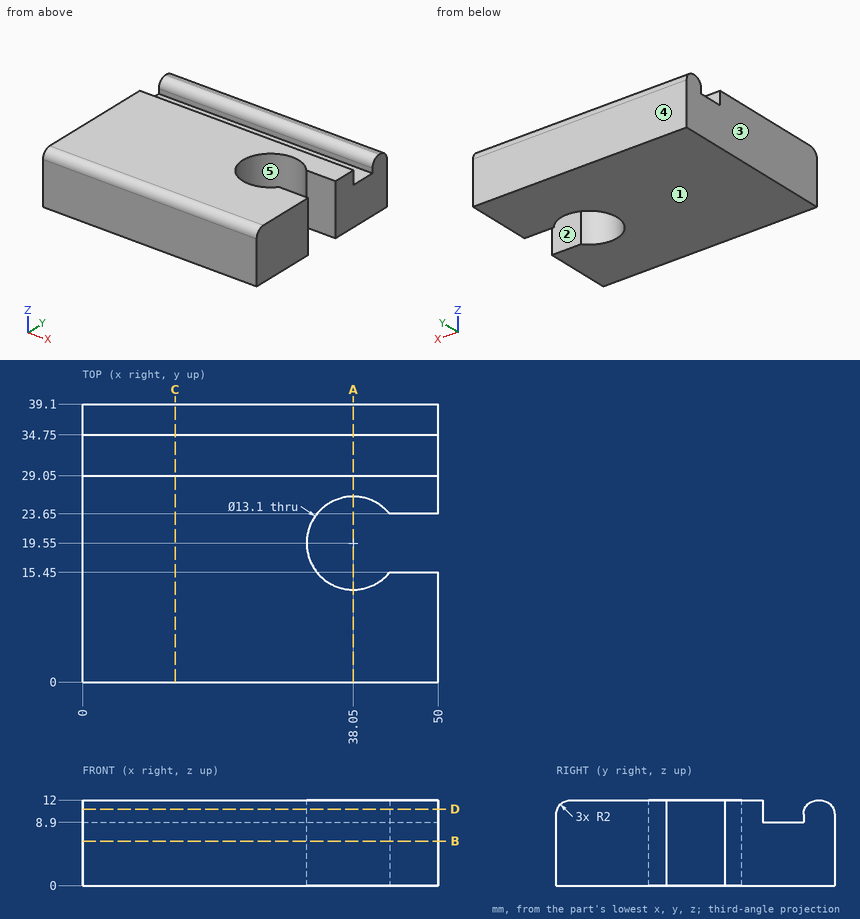
Answer from the drawing. Dimensions are ordinates in mm from the lowest x, y and z of the part. A direction names the side the tool comes from. Round coordinates to 2 decimals unless told otherwise and drop trailing zeros. Loops run counter-clockwise (first coordinate to the right, second up) from the corner with the lowest first, then second, coordinate; pieces in that order, holes last.
1) Given P1, Ø1, axis at x = 8, y = 31, coming from the +Z side, flat-ended and moving along its own axis, determine where the tip first touches the part or whether it passes through.
Outcome:
P1: stops at z = 8.9
2) A cutting plane is placed at C-C on x = 13. Determine the outline of the cut face in (y, z).
Outcome:
outline: (0, 0) - (39.1, 0) - (39.1, 10) arc R2 ccw to (37.1, 12) - (36.75, 12) arc R2 ccw to (34.75, 10) - (34.75, 8.9) - (29.05, 8.9) - (29.05, 12) - (2, 12) arc R2 ccw to (0, 10) - close
3) For the marked faces 1 and 2, determine the directions among +Z, -Z, +X, -X, +Y, -Y from which every point of the face is accessible in a straight line to the end or side of a thin tool.
Outcome:
face 1: -Z, +X, -X, +Y, -Y
face 2: +Z, -Z, +X
4) A cutting plane is placed at D-D on z = 10.75. Determine the outline of the cut face in (x, y).
Outcome:
outline: (0, 0.15) - (50, 0.15) - (50, 15.45) - (43.16, 15.45) arc R6.55 cw (long way) to (43.16, 23.65) - (50, 23.65) - (50, 29.05) - (0, 29.05) - close; (0, 34.9) - (50, 34.9) - (50, 38.95) - (0, 38.95) - close
5) For a pull along X with two mould halves and no side action, classify the marked faces 3, 4 and 5 as released by +X, released by -X, zero draft, split by the parting line, or undercut.
Outcome:
face 3: released by -X
face 4: zero draft
face 5: undercut
6) A cutting plane is placed at A-A on x = 38.05. Determine the outline of the cut face in (y, z).
Outcome:
outline: (0, 0) - (13, 0) - (13, 12) - (2, 12) arc R2 ccw to (0, 10) - close; (26.1, 0) - (39.1, 0) - (39.1, 10) arc R2 ccw to (37.1, 12) - (36.75, 12) arc R2 ccw to (34.75, 10) - (34.75, 8.9) - (29.05, 8.9) - (29.05, 12) - (26.1, 12) - close
7) Consider line 1 (Y direction, x = 38.05, z = 3.5); line 2 (Y direction, x = 27.5, z = 9.75); line 3 (X direction, y = 19.55, z = 3). Determine where each line is inside the solid, lowest interval first.
Outcome:
line 1: y = 0 to 13, 26.1 to 39.1
line 2: y = 0 to 29.05, 34.75 to 39.1
line 3: x = 0 to 31.5
8) A cutting plane is placed at B-B on z = 6.25. Determine the outline of the cut face in (x, y).
Outcome:
outline: (0, 0) - (50, 0) - (50, 15.45) - (43.16, 15.45) arc R6.55 cw (long way) to (43.16, 23.65) - (50, 23.65) - (50, 39.1) - (0, 39.1) - close
